Input: part model. Units: mm. Frame: model coordinates. A direction names the side the tool comes from. Round coordinates to 2 decimals unless told otherwise and drop trailing zeros. Write each loop counter-clockwise with the first axis right and the second up, starting at its lowest first coordinate (ties: lowest second). Pieces come first, ordered by that corner, then holes. Notation, with made-up numbers: (25.5, 62) -> (82.5, 62) arc R22 ccw to (82.5, 82) -> close; hole circle Ø2 at (-3.75, 71). An arc over 180 degrees is marked (long way). Use CSV: the item, a comma, the result in double quotes.
```python
from build123d import *

# Parameters (mm, degrees)
CROQUIS1_R              = 1.5
CROQUIS1_W              = 12.5
CROQUIS1_H              = 63.5
SALIENTE_EXTRUIR1_DEPTH = 15


with BuildPart() as part:
    # Croquis1 → Saliente-Extruir1 (new body)
    with BuildSketch(Plane(origin=(0, 0, 0), x_dir=(1, 0, 0), z_dir=(0, 1, 0))):
        Polygon((-8.25, 33.75), (8.25, 33.75), (8.25, -33.75), (-8.25, -33.75), (-21.25, -33.75), (-21.25, 33.75), align=None)
        with Locations(Location((-13.75, -23.75, 0), (0, 0, 270))):
            Circle(CROQUIS1_R, mode=Mode.SUBTRACT)
        with Locations(Location((-13.75, 23.75, 0), (0, 0, 270))):
            Circle(CROQUIS1_R, mode=Mode.SUBTRACT)
        Rectangle(CROQUIS1_W, CROQUIS1_H, mode=Mode.SUBTRACT)
    extrude(amount=SALIENTE_EXTRUIR1_DEPTH)


solid = part.part
```
Item 1: Section query D-D on x = -1.75. Return the cut outline in (y, z).
Worked answers:
outline,"(0, -33.75) -> (15, -33.75) -> (15, -31.75) -> (0, -31.75) -> close; (0, 31.75) -> (15, 31.75) -> (15, 33.75) -> (0, 33.75) -> close"
Item 2: Section query B-B on y = 1.75. Return the cut outline in (x, z).
Worked answers:
outline,"(-21.25, -33.75) -> (8.25, -33.75) -> (8.25, 33.75) -> (-21.25, 33.75) -> close; hole circle Ø3 at (-13.75, -23.75); hole circle Ø3 at (-13.75, 23.75); hole (-6.25, -31.75) -> (6.25, -31.75) -> (6.25, 31.75) -> (-6.25, 31.75) -> close"
Item 3: Pull-direction query (X, two-part tool) for faces 1 (the face through (-10, 15, 0)), 2 (the face through (0, 7, -31.75)), 3 (the face through (8.25, 7, 0)); classes: +X half, -X half, draft (parallel to the pull), parting line (faces both ways), or undercut.
Worked answers:
face 1,"draft"
face 2,"undercut"
face 3,"+X half"
Item 4: First-contact query: pin 1 Ø1.8 at (x, z) = (-13.75, 23.75) entering from +Y (3 decimals). Flat tip, straight axial feed; report the tip coordinate or a pass-through.
Worked answers:
pin 1,"passes through"
Item 5: Section query C-C on z = -4. Return the cut outline in (x, y).
Worked answers:
outline,"(-21.25, 0) -> (-6.25, 0) -> (-6.25, 15) -> (-21.25, 15) -> close; (6.25, 0) -> (8.25, 0) -> (8.25, 15) -> (6.25, 15) -> close"
Item 6: Set-up query: faces 4 (the face through (-6, 7, -33.75)), 5 (the face through (-6.25, 7, 0)). Return all of +Z, -Z, +X, -X, +Y, -Y with unobstructed straight access to the full face (end or side cutting, diameter ignored); none if empty.
Worked answers:
face 4,"-Z, +X, -X, +Y, -Y"
face 5,"+Y, -Y"
Item 7: Line query: line 1 (X direction, y = 9, z = -23.75); line 2 (Z direction, x = -13.25, y = 11.5); line 3 (X direction, y = 1.75, z = -19.5). Output: solid intervals per line, ascending.
Worked answers:
line 1,"x = -21.25 to -15.25, -12.25 to -6.25, 6.25 to 8.25"
line 2,"z = -33.75 to -25.16, -22.34 to 22.34, 25.16 to 33.75"
line 3,"x = -21.25 to -6.25, 6.25 to 8.25"
Item 8: Section query A-A on x = -13.75. Return the cut outline in (y, z).
Worked answers:
outline,"(0, -33.75) -> (15, -33.75) -> (15, -25.25) -> (0, -25.25) -> close; (0, -22.25) -> (15, -22.25) -> (15, 22.25) -> (0, 22.25) -> close; (0, 25.25) -> (15, 25.25) -> (15, 33.75) -> (0, 33.75) -> close"
